from build123d import *

# Parameters (mm, degrees)
F0_W      = 100
F0_H      = 60
F1_DEPTH  = 50
F2_W      = 70
F2_H      = 15
F3_DEPTH  = 60
F4_W      = 15
F4_H      = 32
F5_DEPTH  = 100
F7_DEPTH  = 50
F9_DEPTH  = 35
F11_DEPTH = 20


with BuildPart() as f1:
    # F0 (on Front) → F1 (new body)
    with BuildSketch(Plane.XZ):
        with Locations((50, 30)):
            Rectangle(F0_W, F0_H)
    extrude(amount=-F1_DEPTH)

    # F2 (on face) → F3 (cut, through all)
    with BuildSketch(Plane.XY.offset(60)):
        with Locations((65, 42.5)):
            Rectangle(F2_W, F2_H)
    extrude(amount=-F3_DEPTH, mode=Mode.SUBTRACT)

    # F4 (on face) → F5 (cut, through all)
    with BuildSketch(Plane.YZ.offset(100)):
        with Locations((7.5, 16)):
            Rectangle(F4_W, F4_H)
    extrude(amount=-F5_DEPTH, mode=Mode.SUBTRACT)

    # F6 (on face) → F7 (cut, through all)
    with BuildSketch(Plane.XZ):
        Polygon((0, 40), (15, 60), (0, 60), align=None)
    extrude(amount=-F7_DEPTH, mode=Mode.SUBTRACT)

    # F8 (on face) → F9 (cut, through all)
    with BuildSketch(Plane.XZ):
        Polygon((100, 60), (55, 60), (86.5, 32), (100, 32), align=None)
    extrude(amount=-F9_DEPTH, mode=Mode.SUBTRACT)

    # F10 (on face) → F11 (cut, through all)
    with BuildSketch(Plane.XZ.offset(-15)):
        Polygon((100, 32), (86.5, 32), (100, 20), align=None)
    extrude(amount=-F11_DEPTH, mode=Mode.SUBTRACT)


solid = f1.part
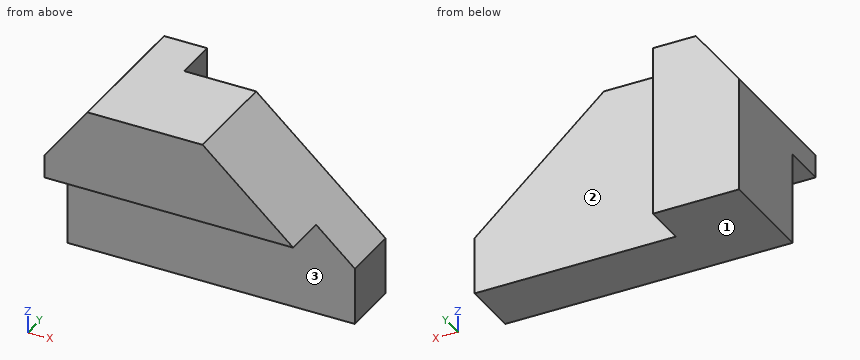
Part model, mm, in its own coordinate system. Face numbers are marked on the shaded views. A direction names the side the tool comes from. Give positions to 0.01 mm unless a question says otherwise; leave off trailing zeros. Order: outer loops, then holes, each group sorted by start corner. A loop starts at its lowest first (then second) coordinate and runs counter-clockwise, first axis right, second up. Notation, with made-up numbers: (-17, 45.25) - (22, 45.25) arc R33 cw to (22, 77.25) - close; hole circle Ø5 at (4.5, -2.5). An arc over 180 degrees is marked (long way). One line per question, with ' | ' between items.
1. Band-saw the part on A-A on x = 17.5. List the corners of the cut face in (y, z), then the cut area to 3 significant figures.
Filled in:
outline: (0, 32) - (15, 32) - (15, 0) - (50, 0) - (50, 60) - (0, 60) - close | area: 2,520 mm²
2. Band-saw the part on D-D on y = 12.5. List the corners of the cut face in (x, z), then the cut area to 3 significant figures.
Filled in:
outline: (0, 32) - (86.5, 32) - (55, 60) - (15, 60) - (0, 40) - close | area: 1,830 mm²
3. Drill centre lines: probe 1 along X at (y, z) = (39, 18.5); probe 2 along Y at (x, z) = (40, 42); probe 3 along Z at (x, y) = (35.5, 4.5). Where is each one in solid material? Low to high.
Filled in:
probe 1: 0 to 30 | probe 2: 0 to 35 | probe 3: 32 to 60
4. Band-saw the part on C-C on z = 56. List the corners of the cut face in (x, y).
Filled in:
outline: (12, 0) - (59.5, 0) - (59.5, 35) - (30, 35) - (30, 50) - (12, 50) - close
5. Band-saw the part on B-B on y = 41.5. List the corners of the cut face in (x, z).
Filled in:
outline: (0, 0) - (30, 0) - (30, 60) - (15, 60) - (0, 40) - close
6. Drop flat-ended pins along their axis: P1, Ø7.5, axis at y = 40.5, z = 31, coming from the +X side; P2, Ø3, axis at y = 23.5, z = 23, coming from the +X side; P3, Ø12, axis at x = 26.5, y = 6, coming from the -Z side. Give the stop position or say it passes through.
Filled in:
P1: x = 30 | P2: x = 98.31 | P3: z = 32
7. Which spindle directions (+Z, -Z, +X, -X, +Y, -Y) get a long thin tool onto all of the face, cutting with end or side? Do the marked faces 1, 2 and 3. Say none if no direction does.
Filled in:
face 1: -Z, +X, -X, +Y, -Y | face 2: +Z, -Z, +X, +Y | face 3: -Z, +X, -X, -Y
